The model under review builds one solid part; all positions refer to its coordinate system, in mm. A direction names the side the tool comes from. Coordinates: 2 decimals unless noted, no trailing zeros. Write each loop counter-clockwise with the first axis right and the second up, starting at its lowest first coordinate (ties: lowest second). Pieces come first, ordered by that corner, then holes. Notation, with made-up numbers: (62.5, 69) - (94.5, 69) arc R23 cw to (94.5, 84) - close; hole circle Ø4 at (53.25, -15). An arc over 180 degrees is marked (long way). Put each result on its own line as item: value.
from build123d import *

# Parameters (mm, degrees)
EXTRUDE_1_DEPTH     = 10
CUT_EXTRUDE_1_DEPTH = 172.090332978
CUT_EXTRUDE_2_DEPTH = 172.0903331
SKETCH_4_R          = 6.822924711
CUT_EXTRUDE_3_DEPTH = 172.0903331
SKETCH_5_R          = 10
CUT_EXTRUDE_4_DEPTH = 172.0903331


with BuildPart() as part:
    # 草图1 → 凸台-拉伸1 (new body)
    with BuildSketch(Plane(origin=(0, 0, 0), x_dir=(1, 0, 0), z_dir=(0, 1, 0))):
        with BuildLine():
            Line((-19.5, 150), (-29.5, 0))
            ThreePointArc((-29.5, 0), (0, -29.5), (29.5, 0))
            Line((29.5, 0), (19.47339908, 150.003410942))
            ThreePointArc((19.47339908, 150.003410942), (-0.014895879, 168.230948441), (-19.5, 150))
        make_face()
    extrude(amount=EXTRUDE_1_DEPTH)

    # 草图2 → 切除-拉伸1 (cut, through all)
    with BuildSketch(Plane(origin=(0, 10, 0), x_dir=(1, 0, 0), z_dir=(0, 1, 0))):
        with BuildLine():
            Line((-18.406498031, 166.402529529), (-29.5, 0))
            add(Edge.make_bspline(
                [(-18.406498031, 166.402529529), (-4.887642604, 82.123380262), (-29.5, 0)],
                knots=[0, 0, 0, 1, 1, 1], degree=2))
        make_face()
        with BuildLine():
            Line((18.377392911, 166.400260194), (29.5, 0))
            add(Edge.make_bspline(
                [(18.377392911, 166.400260194), (6.100316571, 82.176287971), (29.5, 0)],
                knots=[0, 0, 0, 1, 1, 1], degree=2))
        make_face()
    extrude(amount=-CUT_EXTRUDE_1_DEPTH, mode=Mode.SUBTRACT)

    # 草图3 → 切除-拉伸2 (cut, through all)
    with BuildSketch(Plane(origin=(0, 10, 0), x_dir=(1, 0, 0), z_dir=(0, 1, 0))):
        with BuildLine():
            Line((-2.5, 90.215422083), (-2.5, 134.474861862))
            ThreePointArc((-2.5, 134.474861862), (0, 136.974861862), (2.5, 134.474861862))
            Line((2.5, 134.474861862), (2.5, 90.215422083))
            ThreePointArc((2.5, 90.215422083), (0, 87.715422083), (-2.5, 90.215422083))
        make_face()
        with BuildLine():
            Line((2.5, 76.205239707), (2.5, 26.214361684))
            ThreePointArc((2.5, 26.214361684), (0, 23.714361684), (-2.5, 26.214361684))
            Line((-2.5, 26.214361684), (-2.5, 76.205239707))
            ThreePointArc((-2.5, 76.205239707), (0, 78.705239707), (2.5, 76.205239707))
        make_face()
    extrude(amount=-CUT_EXTRUDE_2_DEPTH, mode=Mode.SUBTRACT)

    # 草图4 → 切除-拉伸3 (cut, through all)
    with BuildSketch(Plane(origin=(0, 10, 0), x_dir=(1, 0, 0), z_dir=(0, 1, 0))):
        with Locations(Location((0, 154.809118853, 0), (0, 0, 270))):
            Circle(SKETCH_4_R)
    extrude(amount=-CUT_EXTRUDE_3_DEPTH, mode=Mode.SUBTRACT)

    # 草图5 → 切除-拉伸4 (cut, through all)
    with BuildSketch(Plane(origin=(0, 10, 0), x_dir=(1, 0, 0), z_dir=(0, 1, 0))):
        with Locations(Location((0, 0, 0), (0, 0, 270))):
            Circle(SKETCH_5_R)
    extrude(amount=-CUT_EXTRUDE_4_DEPTH, mode=Mode.SUBTRACT)


solid = part.part
1. To check wall thickness, follow probe 1 along X at (y, z) = (5.5, -58); probe 2 along X at (y, z) = (7.75, -51); probe 3 along X at (y, z) = (2.25, -13). State the ranges of each line that lie inside material, in increasing order.
Determined:
probe 1: x = -16.91 to -2.5, 2.5 to 17.46
probe 2: x = -17.92 to -2.5, 2.5 to 18.44
probe 3: x = -25.85 to 26.02
2. The part is to be moulded in two halves that separate along X. For faces 3 (the cylindrical face through (-0.055, 5.07, -78.705)), 4 (the flat face through (2.5, 5, -52)), 5 (the flat face through (-7, 10, -49)), 6 (the cylindrical face through (-0.649, 4.93, 29.493)), say which applies: +X half, -X half, draft (parallel to the pull), parting line (faces both ways), or undercut.
Determined:
face 3: undercut
face 4: undercut
face 5: draft
face 6: parting line
3. Consider section A-A on x = 0. State the section outline as (y, z) points, plus the area to 3 significant figures.
Determined:
outline: (0, -168.23) - (10, -168.23) - (10, -161.63) - (0, -161.63) - close; (0, -147.99) - (10, -147.99) - (10, -136.97) - (0, -136.97) - close; (0, -87.72) - (10, -87.72) - (10, -78.71) - (0, -78.71) - close; (0, -23.71) - (10, -23.71) - (10, -10) - (0, -10) - close; (0, 10) - (10, 10) - (10, 29.5) - (0, 29.5) - close
area: 598 mm^2
4. Machinability: for faces 1 (the flat face through (-2.5, 5, -51)), 2 (the flat face through (-7, 0, -49)), which of the approach directions +Z, -Z, +X, -X, +Y, -Y give a long, thin tool a straight path to every point of the face, cutting with its end or side? Answer none if there is none.
Determined:
face 1: +Y, -Y
face 2: +Z, -Z, +X, -X, -Y
5. Consider section C-C on z = 18. State the section outline as (x, y) points.
Determined:
outline: (-23.37, 0) - (23.37, 0) - (23.37, 10) - (-23.37, 10) - close
6. For pin 1 Ø5 at (y, z) = (6.5, -51.5) entering from -X; pin 2 Ø23 at (x, z) = (0, 0) entering from +Y; pin 3 Ø3 at (x, y) = (18, 6.5) entering from -Z; pin 4 Ø1 at (y, z) = (6, -100.5) entering from +X, all flat-tipped, find the tip position at first contact; note any pin that passes through.
Determined:
pin 1: stops at x = -18.24
pin 2: stops at y = 10
pin 3: stops at z = -159.13
pin 4: stops at x = 14.25
7. Consider section B-B on y = 7. Give the number of separate pieces and of enclosed holes in the cut face, plus the area to 3 significant figures.
Determined:
separate pieces: 1
enclosed holes: 4
area: 6,260 mm^2
